from build123d import *

# Parameters (mm, degrees)
SKETCH_2_W          = 62.5
SKETCH_2_H          = 3.676470588
EXTRUDE_1_DEPTH     = 40
SKETCH_4_R          = 2
SKETCH_4_R_2        = 5
SKETCH_4_R_3        = 2.5
CUT_EXTRUDE_1_DEPTH = 75.295130634
SKETCH_5_W          = 125
SKETCH_5_H          = 3.676470588
EXTRUDE_3_DEPTH     = 50
SKETCH_6_W          = 130
SKETCH_6_H          = 3.676470588
EXTRUDE_4_DEPTH     = 12
SKETCH_7_R          = 2.5
CUT_EXTRUDE_2_DEPTH = 117.892114516
SKETCH_8_W          = 130
SKETCH_8_H          = 3.676470588
EXTRUDE_5_DEPTH     = 20
CUT_EXTRUDE_4_DEPTH = 131.55177684
SKETCH_11_W         = 130
SKETCH_11_H         = 3.676470588
EXTRUDE_6_DEPTH     = 15
SKETCH_12_W         = 172
SKETCH_12_H         = 3.676470588
EXTRUDE_7_DEPTH     = 20
CUT_EXTRUDE_5_DEPTH = 146.064697415
FILLET_2_R          = 5


with BuildPart() as part:
    # 草图2 → 凸台-拉伸1 (new, symmetric)
    with BuildSketch(Plane.XY):
        with Locations((-31.25, 1.838235294)):
            Rectangle(SKETCH_2_W, SKETCH_2_H)
    extrude_1 = extrude(amount=EXTRUDE_1_DEPTH, both=True)

    # 镜向1: 凸台-拉伸1 across plane
    add(extrude_1.mirror(Plane(origin=(0, 0, 40), x_dir=(0, 0, 1), z_dir=(-1, 0, 0))))

    # 草图4 → 切除-拉伸1 (cut, through all)
    with BuildSketch(Plane(origin=(0, 3.676470588, 0), x_dir=(1, 0, 0), z_dir=(0, 1, 0))):
        with Locations(Location((0, 15.5, 0), (0, 0, 180))):
            Circle(SKETCH_4_R)
        with Locations(Location((15.5, 0, 0), (0, 0, 180))):
            Circle(SKETCH_4_R)
        with Locations(Location((0, -15.5, 0), (0, 0, 180))):
            Circle(SKETCH_4_R)
        with Locations(Location((-15.5, 0, 0), (0, 0, 180))):
            Circle(SKETCH_4_R)
        with Locations(Location((0, 0, 0), (0, 0, 180))):
            Circle(SKETCH_4_R_2)
        with Locations(Location((-52.5, 10, 0), (0, 0, 180))):
            Circle(SKETCH_4_R_3)
        with Locations(Location((-52.5, 30, 0), (0, 0, 180))):
            Circle(SKETCH_4_R_3)
        with Locations(Location((-52.5, -10, 0), (0, 0, 180))):
            Circle(SKETCH_4_R_3)
        with Locations(Location((-52.5, -30, 0), (0, 0, 180))):
            Circle(SKETCH_4_R_3)
    extrude(amount=-CUT_EXTRUDE_1_DEPTH, mode=Mode.SUBTRACT)

    # 草图5 → 凸台-拉伸3 (add)
    with BuildSketch(Plane.XY.offset(40)):
        with Locations((0, 1.838235294)):
            Rectangle(SKETCH_5_W, SKETCH_5_H)
    extrude(amount=EXTRUDE_3_DEPTH)

    # 草图6 → 凸台-拉伸4 (add)
    with BuildSketch(Plane(origin=(62.5, 0, 0), x_dir=(0, 0, -1), z_dir=(1, 0, 0))):
        with Locations((-25, 1.838235294)):
            Rectangle(SKETCH_6_W, SKETCH_6_H)
    extrude(amount=EXTRUDE_4_DEPTH)

    # 草图7 → 切除-拉伸2 (cut, through all)
    with BuildSketch(Plane(origin=(0, 3.676470588, 0), x_dir=(1, 0, 0), z_dir=(0, 1, 0))):
        with Locations(Location((68.5, 30, 0), (0, 0, 180))):
            Circle(SKETCH_7_R)
        with Locations(Location((68.5, 10, 0), (0, 0, 180))):
            Circle(SKETCH_7_R)
        with Locations(Location((68.5, -10, 0), (0, 0, 180))):
            Circle(SKETCH_7_R)
        with Locations(Location((68.5, -30, 0), (0, 0, 180))):
            Circle(SKETCH_7_R)
    extrude(amount=-CUT_EXTRUDE_2_DEPTH, mode=Mode.SUBTRACT)

    # 草图8 → 凸台-拉伸5 (add)
    with BuildSketch(Plane(origin=(74.5, 0, 0), x_dir=(0, 0, -1), z_dir=(1, 0, 0))):
        with Locations((-25, 1.838235294)):
            Rectangle(SKETCH_8_W, SKETCH_8_H)
    extrude(amount=EXTRUDE_5_DEPTH)

    # 草图10 → 切除-拉伸4 (cut, through all)
    with BuildSketch(Plane(origin=(0, 3.676470588, 0), x_dir=(1, 0, 0), z_dir=(0, 1, 0))):
        with BuildLine():
            Line((68.5, 32.5), (83.5, 32.5))
            ThreePointArc((83.5, 32.5), (86, 30), (83.5, 27.5))
            Line((83.5, 27.5), (68.5, 27.5))
            ThreePointArc((68.5, 27.5), (66, 30), (68.5, 32.5))
        make_face()
        with BuildLine():
            Line((68.5, 12.5), (83.5, 12.5))
            ThreePointArc((83.5, 12.5), (86, 10), (83.5, 7.5))
            Line((83.5, 7.5), (68.5, 7.5))
            ThreePointArc((68.5, 7.5), (66, 10), (68.5, 12.5))
        make_face()
        with BuildLine():
            Line((68.5, -7.5), (83.5, -7.5))
            ThreePointArc((83.5, -7.5), (86, -10), (83.5, -12.5))
            Line((83.5, -12.5), (68.5, -12.5))
            ThreePointArc((68.5, -12.5), (66, -10), (68.5, -7.5))
        make_face()
        with BuildLine():
            Line((68.5, -27.5), (83.5, -27.5))
            ThreePointArc((83.5, -27.5), (86, -30), (83.5, -32.5))
            Line((83.5, -32.5), (68.5, -32.5))
            ThreePointArc((68.5, -32.5), (66, -30), (68.5, -27.5))
        make_face()
    extrude(amount=-CUT_EXTRUDE_4_DEPTH, mode=Mode.SUBTRACT)

    # 草图11 → 凸台-拉伸6 (add)
    with BuildSketch(Plane.ZY.offset(62.5)):
        with Locations((25, 1.838235294)):
            Rectangle(SKETCH_11_W, SKETCH_11_H)
    extrude(amount=EXTRUDE_6_DEPTH)

    # 草图12 → 凸台-拉伸7 (add)
    with BuildSketch(Plane.XY.offset(90)):
        with Locations((8.5, 1.838235294)):
            Rectangle(SKETCH_12_W, SKETCH_12_H)
    extrude(amount=EXTRUDE_7_DEPTH)

    # 草图13 → 切除-拉伸5 (cut, through all)
    with BuildSketch(Plane(origin=(0, 3.676470588, 0), x_dir=(1, 0, 0), z_dir=(0, 1, 0))):
        with BuildLine():
            Line((80, -99.512851956), (70, -99.512851956))
            ThreePointArc((70, -99.512851956), (65.5, -95.012851956), (70, -90.512851956))
            Line((70, -90.512851956), (80, -90.512851956))
            ThreePointArc((80, -90.512851956), (84.5, -95.012851956), (80, -99.512851956))
        make_face()
        with BuildLine():
            Line((37.573593129, -99.713203436), (27.573593129, -99.713203436))
            ThreePointArc((27.573593129, -99.713203436), (23.073593129, -95.213203436), (27.573593129, -90.713203436))
            Line((27.573593129, -90.713203436), (37.573593129, -90.713203436))
            ThreePointArc((37.573593129, -90.713203436), (42.073593129, -95.213203436), (37.573593129, -99.713203436))
        make_face()
        with BuildLine():
            Line((37.573593129, -57.286796564), (27.573593129, -57.286796564))
            ThreePointArc((27.573593129, -57.286796564), (23.073593129, -52.786796564), (27.573593129, -48.286796564))
            Line((27.573593129, -48.286796564), (37.573593129, -48.286796564))
            ThreePointArc((37.573593129, -48.286796564), (42.073593129, -52.786796564), (37.573593129, -57.286796564))
        make_face()
        with BuildLine():
            Line((80, -57.520090719), (70, -57.520090719))
            ThreePointArc((70, -57.520090719), (65.266705846, -52.786796564), (70, -48.05350241))
            Line((70, -48.05350241), (80, -48.05350241))
            ThreePointArc((80, -48.05350241), (84.733294154, -52.786796564), (80, -57.520090719))
        make_face()
    extrude(amount=-CUT_EXTRUDE_5_DEPTH, mode=Mode.SUBTRACT)

    # 圆角2
    fillet_2_edges = [part.edges().sort_by_distance(p)[0] for p in [
        (94.5, 1.838235294, -40),
        (-77.5, 1.838235294, -40),
        (94.5, 1.838235294, 110),
        (-77.5, 1.838235294, 110),
    ]]
    fillet(fillet_2_edges, radius=FILLET_2_R)


solid = part.part
Verification items for the finished model (mm, model axes). A direction names the side the tool comes from. Coordinates: 2 decimals unless noted, no trailing zeros. Order: outer loops, then holes, each group sorted by start corner. A loop starts at its lowest first (then second) coordinate and runs counter-clockwise, first axis right, second up. Notation, with made-up numbers: M 60.5,3 L 116.5,3 A28 ccw 116.5,36 Z; hole C 89.25,27 d6. An arc over 180 degrees is marked long. One line per item, written item: value. Start each with the question number.
Item 1: Depth check by flat-ended pin: P1, Ø6, axis at x = 27.5, z = 50.5, coming from the -Y side. Enter the tip coordinate at first touch or a pass-through.
Item 2: Thickness scan on probe 1 along Z at (x, y) = (-52.5, 0.9); probe 2 along Z at (x, y) = (-15.5, 1.2); probe 3 along Z at (x, y) = (0, 1.3). Record the ranges inside material, lowest first.
Item 3: Sectioned sample at D-D on y = 1.6. Give the number of separate pieces and of enclosed holes in the cut face, then the cut area to 3 significant figures.
Item 4: Sectioned sample at A-A on z = 0. Record the cut outline in (x, y), then the cut area to 3 significant figures.
Item 5: Access from +Z, -Z, +X, -X, +Y, -Y to the whole of each face (thin tool, end or side, straight path). Record for faces 1 (the flat face through (75, 2, 57.52)), 2 (the flat face through (7, 3.676, 34)).
Item 6: Sectioned sample at B-B on z = -15.5. Record the cut outline in (x, y), then the cut area to 3 significant figures.
Item 7: Sectioned sample at C-C on z = 93.5. Record the cut outline in (x, y), then the cut area to 3 significant figures.
Item 8: Mould release check, pull along Z, two halves, no side actions. Record for faces 3 (the flat face through (7, 2, 110)), 4 (the flat face through (33, 2, 99.713)), 5 (the cylindrical face through (-76.07, 1.86, -38.5)): pulls with the +Z half, pulls with the -Z half, needs draft (parallel to the pull), parting line crosses it, or undercut.
Calculated:
1. P1: y = 0
2. probe 1: -40 to -32.5, -27.5 to -12.5, -7.5 to 7.5, 12.5 to 27.5, 32.5 to 110
2. probe 2: -40 to -2, 2 to 110
2. probe 3: -40 to -17.5, -13.5 to -5, 5 to 13.5, 17.5 to 110
3. separate pieces: 1
3. enclosed holes: 17
3. area: 24,600 mm^2
4. outline: M -77.5,0 L -17.5,0 L -17.5,3.68 L -77.5,3.68 Z; M -13.5,0 L -5,0 L -5,3.68 L -13.5,3.68 Z; M 5,0 L 13.5,0 L 13.5,3.68 L 5,3.68 Z; M 17.5,0 L 94.5,0 L 94.5,3.68 L 17.5,3.68 Z
4. area: 566 mm^2
5. face 1: +Y, -Y
5. face 2: +Z, -Z, +X, -X, +Y
6. outline: M -77.5,0 L -2,0 L -2,3.68 L -77.5,3.68 Z; M 2,0 L 94.5,0 L 94.5,3.68 L 2,3.68 Z
6. area: 618 mm^2
7. outline: M -77.5,0 L 23.41,0 L 23.41,3.68 L -77.5,3.68 Z; M 41.73,0 L 65.76,0 L 65.76,3.68 L 41.73,3.68 Z; M 84.24,0 L 94.5,0 L 94.5,3.68 L 84.24,3.68 Z
7. area: 497 mm^2
8. face 3: pulls with the +Z half
8. face 4: undercut
8. face 5: pulls with the -Z half
